from build123d import *

# Parameters (mm, degrees)
SKETCH1_W           = 600
SKETCH1_H           = 600
SKETCH1_R           = 4.5
BOSS_EXTRUDE1_DEPTH = 4
CUT_EXTRUDE2_REACH  = 850.538
SKETCH4_R           = 3.25
SKETCH4_3_W         = 50
SKETCH4_3_H         = 6
SKETCH4_3_W_2       = 6
SKETCH4_3_H_2       = 40
BOSS_EXTRUDE2_DEPTH = 35


with BuildPart() as part:
    # Sketch1 → Boss-Extrude1 (new body)
    with BuildSketch(Plane(origin=(0, 0, 0), x_dir=(1, 0, 0), z_dir=(0, 1, 0))):
        with Locations((300, 300)):
            Rectangle(SKETCH1_W, SKETCH1_H)
        with Locations(Location((20, 580, 0), (0, 0, 270))):
            Circle(SKETCH1_R, mode=Mode.SUBTRACT)
        with Locations(Location((580, 580, 0), (0, 0, 270))):
            Circle(SKETCH1_R, mode=Mode.SUBTRACT)
        with Locations(Location((580, 20, 0), (0, 0, 270))):
            Circle(SKETCH1_R, mode=Mode.SUBTRACT)
        with Locations(Location((20, 20, 0), (0, 0, 270))):
            Circle(SKETCH1_R, mode=Mode.SUBTRACT)
    extrude(amount=BOSS_EXTRUDE1_DEPTH)

    # Sketch4 → Cut-Extrude2 (cut, up to next)
    with BuildSketch(Plane(origin=(0, 4, 0), x_dir=(1, 0, 0), z_dir=(0, 1, 0)), mode=Mode.PRIVATE) as cut_extrude2_sk1:
        with Locations(Location((390.25, 544, 0), (0, 0, 270))):
            Circle(SKETCH4_R)
    cut_extrude2_tool1 = extrude(cut_extrude2_sk1.sketch, amount=-CUT_EXTRUDE2_REACH, mode=Mode.PRIVATE) & part.part
    # Sketch4 → Cut-Extrude2 (cut, up to next)
    with BuildSketch(Plane(origin=(0, 4, 0), x_dir=(1, 0, 0), z_dir=(0, 1, 0)), mode=Mode.PRIVATE) as cut_extrude2_sk2:
        with Locations(Location((390.25, 436, 0), (0, 0, 270))):
            Circle(SKETCH4_R)
    cut_extrude2_tool2 = extrude(cut_extrude2_sk2.sketch, amount=-CUT_EXTRUDE2_REACH, mode=Mode.PRIVATE) & part.part
    # Sketch4 → Cut-Extrude2 (cut, up to next)
    with BuildSketch(Plane(origin=(0, 4, 0), x_dir=(1, 0, 0), z_dir=(0, 1, 0)), mode=Mode.PRIVATE) as cut_extrude2_sk3:
        with Locations(Location((548.25, 436, 0), (0, 0, 270))):
            Circle(SKETCH4_R)
    cut_extrude2_tool3 = extrude(cut_extrude2_sk3.sketch, amount=-CUT_EXTRUDE2_REACH, mode=Mode.PRIVATE) & part.part
    # Sketch4 → Cut-Extrude2 (cut, up to next)
    with BuildSketch(Plane(origin=(0, 4, 0), x_dir=(1, 0, 0), z_dir=(0, 1, 0)), mode=Mode.PRIVATE) as cut_extrude2_sk4:
        with Locations(Location((548.25, 544, 0), (0, 0, 270))):
            Circle(SKETCH4_R)
    cut_extrude2_tool4 = extrude(cut_extrude2_sk4.sketch, amount=-CUT_EXTRUDE2_REACH, mode=Mode.PRIVATE) & part.part
    add(cut_extrude2_tool1.solids().sort_by_distance((390.25, 4, -544))[0], mode=Mode.SUBTRACT)
    add(cut_extrude2_tool2.solids().sort_by_distance((390.25, 4, -436))[0], mode=Mode.SUBTRACT)
    add(cut_extrude2_tool3.solids().sort_by_distance((548.25, 4, -436))[0], mode=Mode.SUBTRACT)
    add(cut_extrude2_tool4.solids().sort_by_distance((548.25, 4, -544))[0], mode=Mode.SUBTRACT)

    # Sketch4_3 → Boss-Extrude2 (add)
    with BuildSketch(Plane(origin=(0, 4, 0), x_dir=(1, 0, 0), z_dir=(0, 1, 0))):
        with Locations((469.25, 553)):
            Rectangle(SKETCH4_3_W, SKETCH4_3_H)
        with Locations((381.5, 490)):
            Rectangle(SKETCH4_3_W_2, SKETCH4_3_H_2)
        with Locations((557, 490)):
            Rectangle(SKETCH4_3_W_2, SKETCH4_3_H_2)
        with Locations((469.25, 427)):
            Rectangle(SKETCH4_3_W, SKETCH4_3_H)
    extrude(amount=BOSS_EXTRUDE2_DEPTH)


solid = part.part
The model under review builds one solid part; all positions refer to its coordinate system, in mm. A direction names the side the tool comes from. Round coordinates to 2 decimals unless told otherwise and drop trailing zeros. Order: outer loops, then holes, each group sorted by start corner. A loop starts at its lowest first (then second) coordinate and runs counter-clockwise, first axis right, second up. Notation, with made-up numbers: (-1.75, 71) - (28.25, 71) arc R16 cw to (28.25, 89) - close; hole circle Ø6 at (-23.75, -16). An arc over 180 degrees is marked (long way). Use one line per item in the form item = value.
Q1. Clearance check with flat-ended pins moving along their axes: P1, Ø3, axis at y = 25.5, z = -553, coming from the +X side; P2, Ø4, axis at x = 482.5, z = -289.5, coming from the +Y side; P3, Ø1.8, axis at x = 382.5, y = 20.5, coming from the +Z side. State where each tip first meets the part, or that it passes through.
Response values:
P1 = 494.25
P2 = 4
P3 = -470
Q2. Tool access review of faces 4 (the flat face through (469, 21, -430)), 5 (the flat face through (469, 21, -424)), 6 (the flat face through (469, 21, -556)), 7 (the flat face through (554, 21, -490)), 8 (the flat face through (560, 21, -490)): name each direction out of +Z, -Z, +X, -X, +Y, -Y from which nothing blocks a thin tool from reaching the whole face with its end or side.
Response values:
face_4 = +X, -X, +Y
face_5 = +Z, +X, -X, +Y
face_6 = -Z, +X, -X, +Y
face_7 = +Z, -Z, +Y
face_8 = +Z, -Z, +X, +Y
Q3. To check wall thickness, follow line 1 (X direction, y = 1.65, z = -436); line 2 (X direction, y = 2, z = -20); line 3 (Z direction, x = 580, y = 1). State the ranges of each line that lie inside material, in increasing order.
Response values:
line_1 = 0 to 387, 393.5 to 545, 551.5 to 600
line_2 = 0 to 15.5, 24.5 to 575.5, 584.5 to 600
line_3 = -600 to -584.5, -575.5 to -24.5, -15.5 to 0
Q4. Add section B-B on z = -190. Give the boundary of the cut face in (x, y).
Response values:
outline = (0, 0) - (600, 0) - (600, 4) - (0, 4) - close
Q5. Mouldability with a two-part tool opening along X and no side actions: class faces 1 (the flat face through (469, 21, -550)), 2 (the flat face through (378.5, 21, -490)), 3 (the flat face through (384.5, 21, -490)) as pulls with the +X half, pulls with the -X half, needs draft (parallel to the pull), parting line crosses it, or undercut.
Response values:
face_1 = needs draft
face_2 = pulls with the -X half
face_3 = undercut
Q6. Add section C-C on x = 414. Give the boundary of the cut face in (y, z).
Response values:
outline = (0, -600) - (4, -600) - (4, 0) - (0, 0) - close
Q7. Add section A-A on y = 22.5. Give the boundary of the cut face in (x, z).
Response values:
outline = (378.5, -510) - (384.5, -510) - (384.5, -470) - (378.5, -470) - close; (444.25, -556) - (494.25, -556) - (494.25, -550) - (444.25, -550) - close; (444.25, -430) - (494.25, -430) - (494.25, -424) - (444.25, -424) - close; (554, -510) - (560, -510) - (560, -470) - (554, -470) - close
